```python
from build123d import *

# Parameters (mm, degrees)
SKETCH2_W                = 50.8
SKETCH2_H                = 50.8
BOSS_EXTRUDE1_DEPTH      = 19.05
SHELL1_T                 = -2.54
SKETCH4_R                = 6.4135
SKETCH4_R_2              = 2.8575
CUT_EXTRUDE1_DEPTH       = 6.35
SKETCH5_W                = 6.35
SKETCH5_H                = 6.35
BOSS_EXTRUDE3_DEPTH      = 50.8
SKETCH6_R                = 2.2225
CUT_EXTRUDE2_DEPTH       = 51.8
SKETCH7_W                = 10.16
SKETCH7_H                = 6.35
CUT_EXTRUDE3_DEPTH       = 6.35
FILLET1_R                = 3.175
SKETCH8_R                = 6.4135
CUT_EXTRUDE4_DEPTH       = 6.35
SKETCH9_W                = 44.45
SKETCH9_H                = 50.8
SKETCH9_R                = 6.4135
BOSS_EXTRUDE4_DEPTH      = 6.35
BOSS_EXTRUDE4_DEPTH_BACK = 6.35


with BuildPart() as part:
    # Sketch2 → Boss-Extrude1 (new body)
    with BuildSketch(Plane(origin=(0, 0, 0), x_dir=(1, 0, 0), z_dir=(0, 1, 0))):
        with Locations((25.4, 25.4)):
            Rectangle(SKETCH2_W, SKETCH2_H)
    extrude(amount=BOSS_EXTRUDE1_DEPTH)

    # Shell1
    shell1_openings = [part.faces().sort_by_distance(p)[0] for p in [
        (25.4, 9.525, -50.8),
        (25.4, 9.525, 0),
    ]]
    offset(amount=SHELL1_T, openings=shell1_openings, kind=Kind.INTERSECTION)

    # Sketch4 → Cut-Extrude1 (cut)
    with BuildSketch(Plane(origin=(0, 19.05, 0), x_dir=(1, 0, 0), z_dir=(0, 1, 0))):
        with Locations((25.4, 25.4)):
            Circle(SKETCH4_R)
        with Locations((4.064, 46.736)):
            Circle(SKETCH4_R_2)
        with Locations((46.736, 46.736)):
            Circle(SKETCH4_R_2)
        with Locations((46.736, 4.064)):
            Circle(SKETCH4_R_2)
        with Locations((4.064, 4.064)):
            Circle(SKETCH4_R_2)
    extrude(amount=-CUT_EXTRUDE1_DEPTH, mode=Mode.SUBTRACT)

    # Sketch5 → Boss-Extrude3 (add)
    with BuildSketch(Plane.XY):
        with Locations((47.625, 3.175)):
            Rectangle(SKETCH5_W, SKETCH5_H)
    extrude(amount=-BOSS_EXTRUDE3_DEPTH)

    # Sketch6 → Cut-Extrude2 (cut, through all)
    with BuildSketch(Plane.XY):
        with Locations((47.625, 3.175)):
            Circle(SKETCH6_R)
    extrude(amount=-CUT_EXTRUDE2_DEPTH, mode=Mode.SUBTRACT)

    # Sketch7 → Cut-Extrude3 (cut)
    with BuildSketch(Plane(origin=(50.8, 0, 0), x_dir=(0, 0, -1), z_dir=(1, 0, 0))):
        with Locations((15.24, 3.175)):
            Rectangle(SKETCH7_W, SKETCH7_H)
        with Locations((35.56, 3.175)):
            Rectangle(SKETCH7_W, SKETCH7_H)
    extrude(amount=-CUT_EXTRUDE3_DEPTH, mode=Mode.SUBTRACT)

    # Fillet1
    fillet1_edges = [part.edges().sort_by_distance(p)[0] for p in [
        (50.8, 0, -25.4),
        (50.8, 0, -45.72),
        (50.8, 0, -5.08),
    ]]
    fillet(fillet1_edges, radius=FILLET1_R)

    # Sketch8 → Cut-Extrude4 (cut)
    with BuildSketch(Plane(origin=(0, 2.54, 0), x_dir=(1, 0, 0), z_dir=(0, 1, 0))):
        with Locations((25.4, 25.4)):
            Circle(SKETCH8_R)
    extrude(amount=-CUT_EXTRUDE4_DEPTH, mode=Mode.SUBTRACT)

    # Sketch9 → Boss-Extrude4 (add, two sides)
    with BuildSketch(Plane.XZ) as boss_extrude4_sk:
        with Locations((22.225, -25.4)):
            Rectangle(SKETCH9_W, SKETCH9_H)
        with Locations((25.4, -25.4)):
            Circle(SKETCH9_R, mode=Mode.SUBTRACT)
    extrude(amount=BOSS_EXTRUDE4_DEPTH)
    extrude(boss_extrude4_sk.sketch, amount=-BOSS_EXTRUDE4_DEPTH_BACK)


solid = part.part
```
Geometry: final body of the model. Coordinates: model frame, mm. A direction names the side the tool comes from. Coordinates: 2 decimals unless noted, no trailing zeros. Order: outer loops, then holes, each group sorted by start corner. A loop starts at its lowest first (then second) coordinate and runs counter-clockwise, first axis right, second up. Notation, with made-up numbers: (61.5, 32.5) -> (87.5, 32.5) arc R19 ccw to (87.5, 44.5) -> close; hole circle Ø4 at (39, -11.75). An arc over 180 degrees is marked (long way). Use CSV: the item, a comma, the result in double quotes.
1) Line query: line 1 (X direction, y = 17.75, z = -46.5); line 2 (Y direction, x = 39, z = -19); line 3 (X direction, y = 6.5, z = -21). Output: solid intervals per line, ascending.
Findings:
line 1,"x = 0 to 1.22, 6.91 to 43.89, 49.58 to 50.8"
line 2,"y = -6.35 to 6.35, 16.51 to 19.05"
line 3,"x = 0 to 2.54, 48.26 to 50.8"
2) Pin query (flat end, axial travel): pin 1 Ø1.3 at (x, z) = (50, -16) entering from -Y; pin 2 Ø1 at (x, z) = (47, -5.5) entering from -Y; pin 3 Ø1.1 at (x, z) = (2, -47) entering from +Y. Return the tip coordinate at first contact, or that it passes through.
Findings:
pin 1,"stops at y = 6.35"
pin 2,"stops at y = 0"
pin 3,"stops at y = 12.7"
3) Section D-D on x = 25.4. Output: boundary loops of the cut face in (y, z).
Findings:
outline,"(-6.35, -50.8) -> (6.35, -50.8) -> (6.35, -31.81) -> (-6.35, -31.81) -> close; (-6.35, -18.99) -> (6.35, -18.99) -> (6.35, 0) -> (-6.35, 0) -> close; (16.51, -50.8) -> (19.05, -50.8) -> (19.05, -31.81) -> (16.51, -31.81) -> close; (16.51, -18.99) -> (19.05, -18.99) -> (19.05, 0) -> (16.51, 0) -> close"
4) Mould query, pull axis Z, two halves, no side actions, for faces 4 (the flat face through (19, 4, -50.8)), 5 (the cylindrical face through (1.21, 16.63, -4.19)), 6 (the cylindrical face through (49.85, 0.91, -5.15)). Classes: +Z half, -Z half, draft (parallel to the pull), parting line (faces both ways), or undercut.
Findings:
face 4,"-Z half"
face 5,"undercut"
face 6,"draft"
5) Section B-B on x = 38. Output: boundary loops of the cut face in (y, z).
Findings:
outline,"(-6.35, -50.8) -> (6.35, -50.8) -> (6.35, 0) -> (-6.35, 0) -> close; (16.51, -50.8) -> (19.05, -50.8) -> (19.05, 0) -> (16.51, 0) -> close"
6) Section A-A on z = -25.4. State how many separate pieces and enclosed holes the cut face has, then the cut area to 3 significant figures.
Findings:
separate pieces,"2"
enclosed holes,"1"
area,"572 mm^2"
7) Access query for faces 1 (the flat face through (50, 6.35, -35)), 2 (the flat face through (46, 0, -46)), 3 (the flat face through (2.54, 11, -25)). Directions: +Z, -Z, +X, -X, +Y, -Y. A direction counts if a zero-diameter tool reaches every point of the face in a straight line with its end or side. Return the directions, or none.
Findings:
face 1,"+X, -Y"
face 2,"+Z, -Z, +X, -Y"
face 3,"+Z, -Z"
8) Section C-C on y = 8. Output: boundary loops of the cut face in (x, z), then the cut area to 3 significant figures.
Findings:
outline,"(0, -50.8) -> (2.54, -50.8) -> (2.54, 0) -> (0, 0) -> close; (48.26, -50.8) -> (50.8, -50.8) -> (50.8, 0) -> (48.26, 0) -> close"
area,"258 mm^2"
